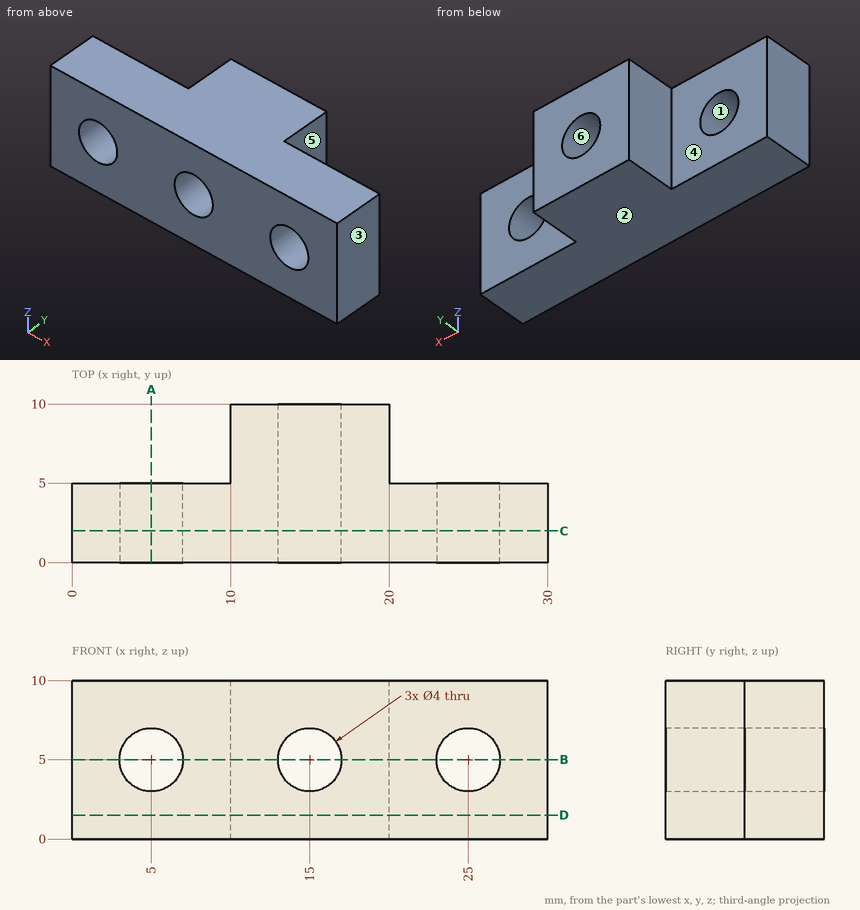
The drawing under review shows one solid part. Ordinate dimensions are in mm from its lowest x, y, z. A direction names the side the tool comes from. Give positions to 0.01 mm unless a question says otherwise; leave off trailing zeros. Write each loop counter-clockwise with the first axis right and the second up, starting at its lowest first coordinate (ties: lowest second). Pieces come first, ordered by that corner, then holes. Notation, with made-up numbers: M 73,64 L 115,64 A36 ccw 115,99 Z; hole C 67.25,-17.75 d3. An arc over 180 degrees is marked long. Write each question's results on one line, items separated by ' | '. Start each with the question number.
1. Mouldability with a two-part tool opening along X and no side actions: class the marked faces 1, 2 and 3 as released by +X, released by -X, zero draft, split by the parting line, or undercut.
2. We need section A-A (x = 5). Write out the cut boundary in (y, z), and give its area (3 significant figures).
3. For probe 1 along Z at (x, y) = (25, 2.55); probe 2 along Y at (x, z) = (9, 8); probe 3 along X at (y, z) = (3.5, 3.5), list the stretches that pass through material, from the lowest coordinate up. Write a range as [from, to].
4. We need section D-D (z = 1.5). Write out the cut boundary in (x, y).
5. We need section C-C (y = 2). Write out the cut boundary in (x, z), and give its area (3 significant figures).
6. For the marked faces 4, 5 and 6, list the 3-axis set-ups (+Z, -Z, +X, -X, +Y, -Y) from which the entire face can be reached by the end or side of a thin tool; tool diameter is ignored.
7. We need section B-B (z = 5). Write out the cut boundary in (x, y).
8. Insertion check: pin 1 Ø2.5 at (y, z) = (8, 6) entering from +X. The pin has a flat end and moves straight along its axis. Give the tip position at first contact, or say it passes through.
Results found:
1) face 1: undercut | face 2: zero draft | face 3: released by +X
2) outline: M 0,0 L 5,0 L 5,3 L 0,3 Z; M 0,7 L 5,7 L 5,10 L 0,10 Z | area: 30.0 mm^2
3) probe 1: z = [0, 3], [7, 10] | probe 2: y = [0, 5] | probe 3: x = [0, 3.68], [6.32, 13.68], [16.32, 23.68], [26.32, 30]
4) outline: M 0,0 L 30,0 L 30,5 L 20,5 L 20,10 L 10,10 L 10,5 L 0,5 Z
5) outline: M 0,0 L 30,0 L 30,10 L 0,10 Z; hole C 5,5 d4; hole C 15,5 d4; hole C 25,5 d4 | area: 262 mm^2
6) face 4: +Z, -Z, -X, +Y | face 5: +Z, -Z, +X, +Y | face 6: +Y, -Y
7) outline: M 0,0 L 3,0 L 3,5 L 0,5 Z; M 7,0 L 13,0 L 13,10 L 10,10 L 10,5 L 7,5 Z; M 17,0 L 23,0 L 23,5 L 20,5 L 20,10 L 17,10 Z; M 27,0 L 30,0 L 30,5 L 27,5 Z
8) pin 1: stops at x = 20
